Verification items for this drawing (mm, ordinates from the low corner). A direction names the side the tool comes from. Round coordinates to 2 decimals unless told otherwise and drop trailing zeros. Loops run counter-clockwise (first coordinate to the right, second up) from the corner with the lowest first, then second, coordinate; pieces in that order, holes last. Notation, with made-up numbers: M -15,19 L 23,19 A15 cw 23,43 Z; hole C -30,-25 d3. An arc over 180 degrees is marked long. Write item = value, one per line. Start each with the question number.
(1) Go/stop test with flat-tipped pins: P1, Ø1.5, axis at y = 15, z = 3.5, coming from the +X side; P2, Ø3, axis at y = 28.5, z = 42, coming from the +X side; P3, Ø5.5, axis at x = 28.5, z = 3, coming from the +Y side; P4, Ø1.5, axis at x = 26.5, y = 15, coming from the +Z side. Record where each tip stops, or that it passes through.
(2) Cross-section at C-C on x = 58. Record the boundary of the cut face in (y, z).
(3) Set-up check for the marked faces 1, 2 and 3: record each of +Z, -Z, +X, -X, +Y, -Y from which the full face is reachable in a straight line by a thin tool's end or side.
(4) Scan lines: L1, parallel to X at y = 23.5, z = 6.5; L2, parallel to Y at x = 39.5, z = 9; L3, parallel to Z at x = 26.5, y = 7. Record each from-to range of solid material in increasing order. Write a range as from..to.
(5) Cross-section at A-A on z = 50. Record the boundary of the cut face in (x, y), plus the area to 3 significant figures.
(6) Cross-section at B-B on x = 30.5. Record the boundary of the cut face in (y, z), plus the area to 3 significant figures.
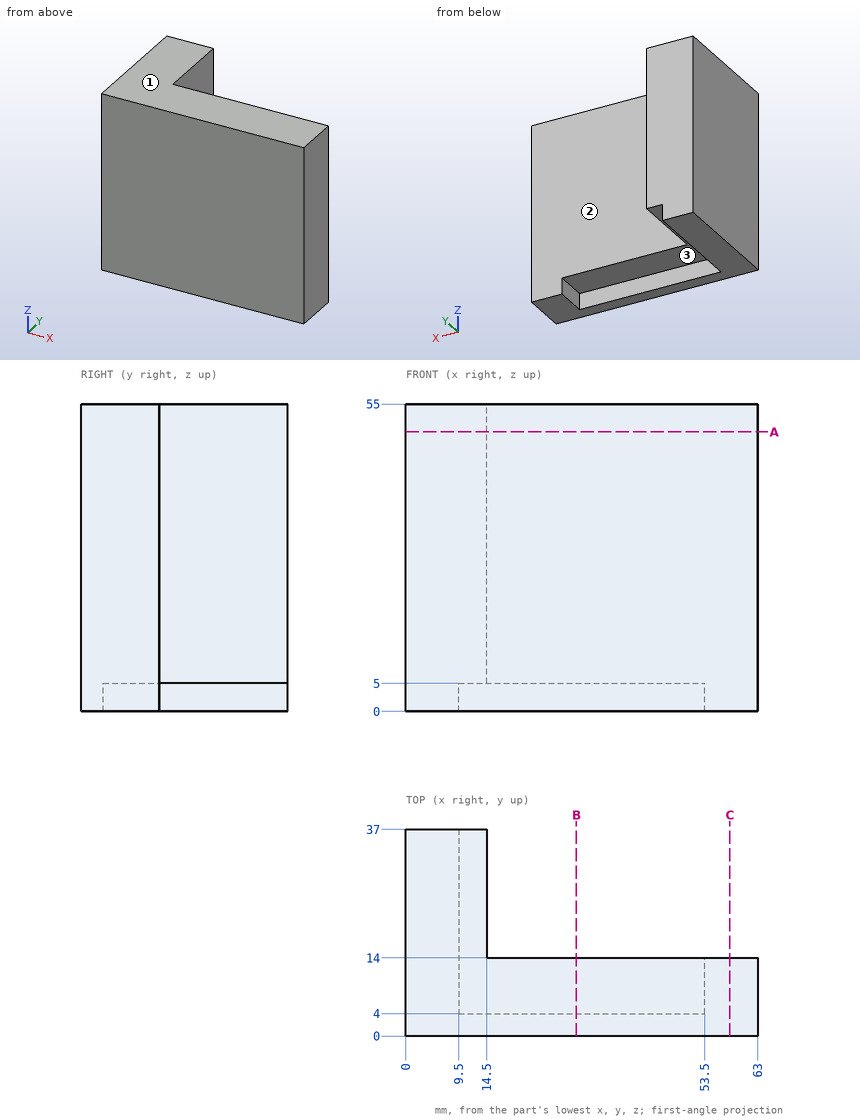
Result:
q1.P1 = 9.5
q1.P2 = 14.5
q1.P3 = 14
q1.P4 = through
q2.outline = M 0,0 L 14,0 L 14,55 L 0,55 Z
q3.face_1 = +Z, +X, -X, +Y, -Y
q3.face_2 = +Z, -Z, +X, +Y
q3.face_3 = -Z, +Y
q4.L1 = 0..14.5
q4.L2 = 0..14
q4.L3 = 5..55
q5.outline = M 0,0 L 63,0 L 63,14 L 14.5,14 L 14.5,37 L 0,37 Z
q5.area = 1,220 mm^2
q6.outline = M 0,0 L 4,0 L 4,5 L 14,5 L 14,55 L 0,55 Z
q6.area = 720 mm^2
